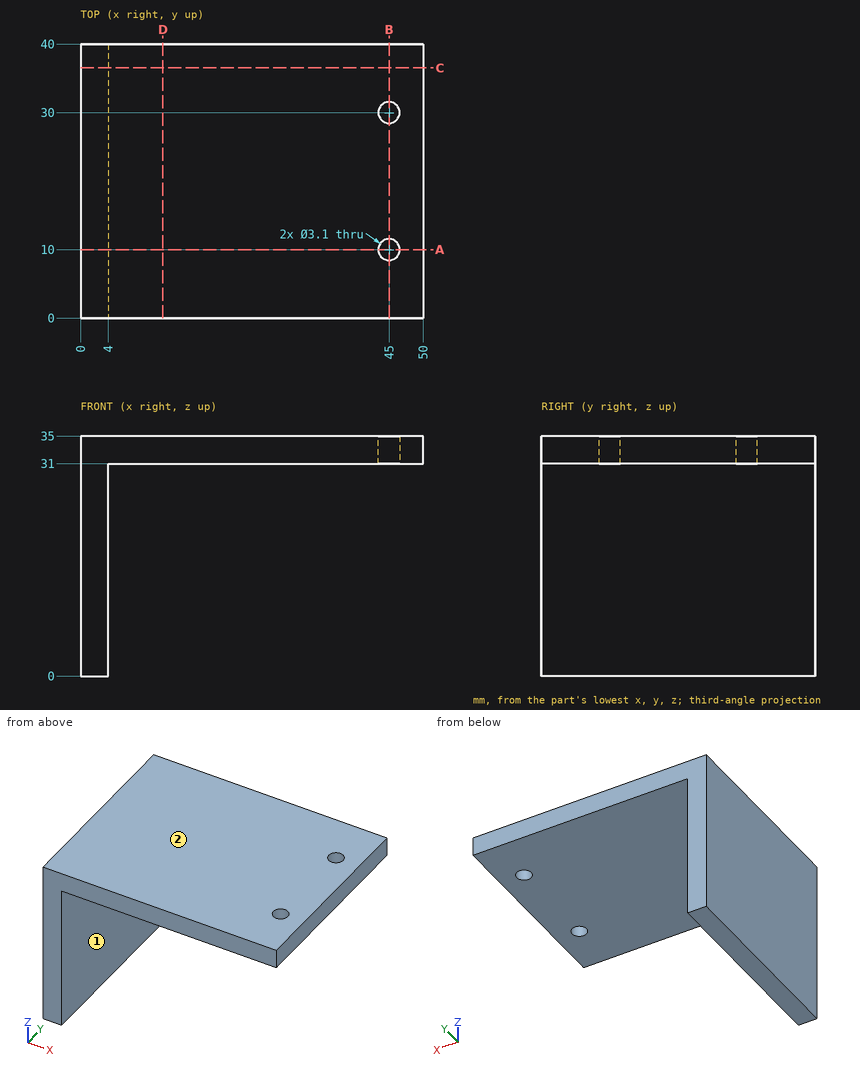
Drawing for the job (mm, zero at the part's lowest x, y, z). A direction names the side the tool comes from. Give positions to 0.01 mm unless a question says otherwise; leave off trailing zeros. Order: outer loops, then holes, each group sorted by start corner. A loop starts at its lowest first (then second) coordinate and runs counter-clockwise, first axis right, second up. Notation, with made-up numbers: M 19,35 L 73,35 A32 cw 73,65 Z; hole C 49,46 d1. An arc over 180 degrees is marked long. Write item = value, one per line. Start each with the question number.
(1) Pin check, flat tips, straight feed: pin 1 Ø4 at (y, z) = (28.5, 14) entering from +X; pin 2 Ø5 at (x, y) = (45, 10) entering from -Z. Stop position of each tip, or through.
(2) Probe L1, parallel to Y at x = 45, z = 32; L2, parallel to X at y = 36, z = 13.5; L3, parallel to Z at x = 10, y = 7.5. List the from-to ranges inside material, lowest first. Write a range as [from, to].
(3) Which spindle directions (+Z, -Z, +X, -X, +Y, -Y) get a long thin tool onto all of the face, cutting with end or side? Do the marked faces 1 and 2. Say none if no direction does.
(4) Slice it at A-A on y = 10. Write the cut outline in (x, z).
(5) Slice it at D-D on x = 12. Write the cut outline in (y, z).
(6) Slice it at C-C on y = 36.5. Write the cut outline in (x, z), plus the area to 3 significant figures.
(7) Slice it at B-B on x = 45. Write the cut outline in (y, z).
Responses:
q1.pin_1 = 4
q1.pin_2 = 31
q2.L1 = [0, 8.45], [11.55, 28.45], [31.55, 40]
q2.L2 = [0, 4]
q2.L3 = [31, 35]
q3.face_1 = -Z, +X, +Y, -Y
q3.face_2 = +Z, +X, -X, +Y, -Y
q4.outline = M 0,0 L 4,0 L 4,31 L 43.45,31 L 43.45,35 L 0,35 Z; M 46.55,31 L 50,31 L 50,35 L 46.55,35 Z
q5.outline = M 0,31 L 40,31 L 40,35 L 0,35 Z
q6.outline = M 0,0 L 4,0 L 4,31 L 50,31 L 50,35 L 0,35 Z
q6.area = 324 mm2
q7.outline = M 0,31 L 8.45,31 L 8.45,35 L 0,35 Z; M 11.55,31 L 28.45,31 L 28.45,35 L 11.55,35 Z; M 31.55,31 L 40,31 L 40,35 L 31.55,35 Z
